```python
from build123d import *

# Parameters (mm, degrees)
SALIENTE_EXTRUIR1_DEPTH = 203.2
SALIENTE_EXTRUIR2_DEPTH = 127


with BuildPart() as part:
    # Croquis1 → Saliente-Extruir1 (new body)
    with BuildSketch(Plane.XY):
        with BuildLine():
            Line((0, 0), (76.2, 0))
            ThreePointArc((76.2, 0), (0, 76.2), (-76.2, 0))
            Line((-76.2, 0), (0, 0))
        make_face()
    extrude(amount=SALIENTE_EXTRUIR1_DEPTH)

    # Croquis2 → Saliente-Extruir2 (add)
    with BuildSketch(Plane.XY.offset(203.2)):
        with BuildLine():
            ThreePointArc((0, 57.15), (-19.05, 38.1), (0, 19.05))
            Line((0, 19.05), (0, 57.15))
        make_face()
        with BuildLine():
            Line((0, 57.15), (0, 19.05))
            ThreePointArc((0, 19.05), (13.470384182, 24.629615818), (19.05, 38.1))
            ThreePointArc((19.05, 38.1), (13.470384182, 51.570384182), (0, 57.15))
        make_face()
    extrude(amount=SALIENTE_EXTRUIR2_DEPTH)


solid = part.part
```
CAD build for the part. Positions are in the model's coordinates, mm. A direction names the side the tool comes from. Coordinates: 2 decimals unless noted, no trailing zeros. Order: outer loops, then holes, each group sorted by start corner. A loop starts at its lowest first (then second) coordinate and runs counter-clockwise, first axis right, second up. Notation, with made-up numbers: M 88.25,-40 L 100.25,-40 A25 cw 100.25,-19 Z; hole C 21,51 d2. An arc over 180 degrees is marked long. Write each question's results on one line, items separated by ' | '. Start each with the question number.
Q1. Cut at B-B (y = 50.5). List the corners of the cut face in (x, z).
Q2. Flat gauge pins, fed straight in: P1, Ø5, axis at y = 57.5, z = 250.5, coming from the +X side; P2, Ø6, axis at x = -31, z = 127.5, coming from the +Y side; P3, Ø23, axis at x = -29.5, y = 48.5, coming from the +Z side. Where does each tip first touch, or does it go through?
Q3. Cut at C-C (x = -37). List the corners of the cut face in (y, z), then the cut area to 3 significant figures.
Q4. Cut at D-D (z = 234). List the corners of the cut face in (x, y).
Q5. Drill centre lines: probe 1 along Z at (x, y) = (-51.5, 33.5); probe 2 along Y at (x, z) = (-26.5, 198.5); probe 3 along X at (y, z) = (31, 105). Where is each one in solid material? Low to high. Write a range as from..to.
Q6. Cut at A-A (z = 176). List the corners of the cut face in (x, y).
Q7. Which spindle directions (+Z, -Z, +X, -X, +Y, -Y) get a long thin tool onto all of the face, cutting with end or side? Do faces 1 (the flat face through (0, 38, 330.2)), 2 (the flat face through (-18, 30, 203.2)). Say none if no direction does.
Found:
1) outline: M -57.06,0 L 57.06,0 L 57.06,203.2 L 14.46,203.2 L 14.46,330.2 L -14.46,330.2 L -14.46,203.2 L -57.06,203.2 Z
2) P1: x = 8.79 | P2: y = 70.87 | P3: z = 203.2
3) outline: M 0,0 L 66.61,0 L 66.61,203.2 L 0,203.2 Z | area: 13,500 mm²
4) outline: C 0,38.1 d38.1
5) probe 1: 0..203.2 | probe 2: 0..71.44 | probe 3: -69.61..69.61
6) outline: M -76.2,0 L 76.2,0 A76.2 ccw Z
7) face 1: +Z, +X, -X, +Y, -Y | face 2: +Z
